The listing builds one solid part. Answer for the finished solid, in the listing's coordinates (mm). A direction names the side the tool comes from. Round coordinates to 2 decimals unless told otherwise and drop trailing zeros. Order: outer loops, then holes, each group sorted by start corner. A loop starts at its lowest first (then second) coordinate and runs counter-clockwise, first axis right, second up. Notation, with made-up numbers: (-39.5, 25.25) - (-27.5, 25.25) arc R15 ccw to (-27.5, 51.25) - close; hole circle Ø10 at (-4, 86). An arc over 180 degrees is marked (long way). Write item = value, one per line.
from build123d import *

# Parameters (mm, degrees)
BOSS_EXTRUDE1_DEPTH = 11
SKETCH2_R           = 35
CUT_EXTRUDE1_DEPTH  = 20
SKETCH3_R           = 14
BOSS_EXTRUDE2_DEPTH = 5
SKETCH4_R           = 10
CUT_EXTRUDE2_DEPTH  = 55
FILLET1_R           = 4
CHAMFER1_SIZE       = 2
SKETCH5_R           = 4
CUT_EXTRUDE3_DEPTH  = 10
SKETCH6_R           = 4
CUT_EXTRUDE4_DEPTH  = 31
SKETCH7_R           = 3
CUT_EXTRUDE5_DEPTH  = 6


with BuildPart() as part:
    # Sketch1 → Boss-Extrude1 (new body, symmetric)
    with BuildSketch(Plane.XY):
        with BuildLine():
            Line((-51.041834152, 0), (51.041834152, 0))
            Line((51.041834152, 0), (51.041834152, 10))
            Line((51.041834152, 10), (37, 10))
            ThreePointArc((37, 10), (34.171572875, 11.171572875), (33, 14))
            Line((33, 14), (33, 21.326056007))
            ThreePointArc((33, 21.326056007), (33.651668366, 24.876928527), (35.52173913, 27.965002788))
            ThreePointArc((35.52173913, 27.965002788), (47.48845464, 58.45277704), (36.877361169, 89.438440728))
            ThreePointArc((36.877361169, 89.438440728), (35.216671351, 92.397361701), (34.641016151, 95.741270355))
            Line((34.641016151, 95.741270355), (34.641016151, 107))
            Line((34.641016151, 107), (0, 107))
            ThreePointArc((0, 107), (-43.325294965, 78.972257605), (-35.52173913, 27.965002788))
            ThreePointArc((-35.52173913, 27.965002788), (-33.651668366, 24.876928527), (-33, 21.326056007))
            Line((-33, 21.326056007), (-33, 14))
            ThreePointArc((-33, 14), (-34.171572875, 11.171572875), (-37, 10))
            Line((-37, 10), (-51.041834152, 10))
            Line((-51.041834152, 10), (-51.041834152, 0))
        make_face()
    extrude(amount=BOSS_EXTRUDE1_DEPTH, both=True)

    # Sketch2 → Cut-Extrude1 (cut)
    with BuildSketch(Plane.XY.offset(11)):
        with Locations((0, 59.5)):
            Circle(SKETCH2_R)
    extrude(amount=-CUT_EXTRUDE1_DEPTH, mode=Mode.SUBTRACT)

    # Sketch3 → Boss-Extrude2 (add)
    with BuildSketch(Plane(origin=(0, 0, -11), x_dir=(-1, 0, 0), z_dir=(0, 0, -1))):
        with Locations((0, 59.5)):
            Circle(SKETCH3_R)
    extrude(amount=BOSS_EXTRUDE2_DEPTH)

    # Sketch4 → Cut-Extrude2 (cut)
    with BuildSketch(Plane(origin=(0, 0, -16), x_dir=(-1, 0, 0), z_dir=(0, 0, -1))):
        with Locations((0, 59.5)):
            Circle(SKETCH4_R)
    extrude(amount=-CUT_EXTRUDE2_DEPTH, mode=Mode.SUBTRACT)

    # Fillet1
    fillet1_edges = [part.edges().sort_by_distance(p)[0] for p in [
        (14, 59.5, -11),
    ]]
    fillet(fillet1_edges, radius=FILLET1_R)

    # Chamfer1
    chamfer1_edges = [part.edges().sort_by_distance(p)[0] for p in [
        (-51.041834152, 5, -11),
        (51.041834152, 5, -11),
        (51.041834152, 5, 11),
        (-51.041834152, 5, 11),
    ]]
    chamfer(chamfer1_edges, length=CHAMFER1_SIZE)

    # Sketch5 → Cut-Extrude3 (cut)
    with BuildSketch(Plane(origin=(0, 10, 0), x_dir=(1, 0, 0), z_dir=(0, 1, 0))):
        with Locations((-42, 0)):
            Circle(SKETCH5_R)
        with Locations((42, 0)):
            Circle(SKETCH5_R)
    extrude(amount=-CUT_EXTRUDE3_DEPTH, mode=Mode.SUBTRACT)

    # Sketch6 → Cut-Extrude4 (cut)
    with BuildSketch(Plane(origin=(0, 107, 0), x_dir=(1, 0, 0), z_dir=(0, 1, 0))):
        with Locations((26.861016151, 0)):
            Circle(SKETCH6_R)
    extrude(amount=-CUT_EXTRUDE4_DEPTH, mode=Mode.SUBTRACT)

    # Sketch7 → Cut-Extrude5 (cut)
    with BuildSketch(Plane.XY.offset(11)):
        with Locations((0, 99.5)):
            Circle(SKETCH7_R)
        with Locations((34.641016151, 79.5)):
            Circle(SKETCH7_R)
        with Locations((34.641016151, 39.5)):
            Circle(SKETCH7_R)
        with Locations((0, 19.5)):
            Circle(SKETCH7_R)
        with Locations((-34.641016151, 39.5)):
            Circle(SKETCH7_R)
        with Locations((-34.641016151, 79.5)):
            Circle(SKETCH7_R)
    extrude(amount=-CUT_EXTRUDE5_DEPTH, mode=Mode.SUBTRACT)


solid = part.part
Q1. Section B-B on z = 0 is taken. Determine the outline of the cut face in (x, y) (3 decimals), then the cut area to 3 significant figures.
Model answer:
outline = (-51.042, 0) - (-46, 0) - (-46, 10) - (-51.042, 10) - close; (-38, 0) - (38, 0) - (38, 10) - (37, 10) arc R4 cw to (33, 14) - (33, 21.326) arc R10 cw to (35.522, 27.965) arc R47.5 ccw to (36.877, 89.438) arc R10 cw to (34.641, 95.741) - (34.641, 107) - (30.861, 107) - (30.861, 76.011) arc R35 cw (long way) to (22.861, 86.002) - (22.861, 107) - (0, 107) arc R47.5 ccw to (-35.522, 27.965) arc R10 cw to (-33, 21.326) - (-33, 14) arc R4 cw to (-37, 10) - (-38, 10) - close; (46, 0) - (51.042, 0) - (51.042, 10) - (46, 10) - close
area = 4,480 mm^2
Q2. For faces 1 (the face through (10, 42, -11)), 2 (the face through (-33, 18, 0)), 3 (the face through (-35, 80, 5)), determine the directions among +Z, -Z, +X, -X, +Y, -Y from which every point of the face is accessible in a straight line to the end or side of a thin tool.
Model answer:
face_1 = -Z
face_2 = +Z, -Z, -X
face_3 = +Z
Q3. Section C-C on x = -42 is taken. Determine the outline of the cut face in (y, z).
Model answer:
outline = (0, -11) - (10, -11) - (10, -4) - (0, -4) - close; (0, 4) - (10, 4) - (10, 11) - (0, 11) - close; (37.31, -11) - (81.69, -11) - (81.69, 11) - (37.31, 11) - close
Q4. Flat-ended cylindrical pins translate along their axes: P1, Ø1.8, axis at x = 1, y = 100, coming from the +Z side; P2, Ø5.5, axis at x = 34.64, y = 39.5, coming from the -Z side; P3, Ø6, axis at x = -30, z = -3.5, coming from the +Y side; P4, Ø5, axis at x = 34, y = 38.5, coming from the +Z side. Find the tip coordinate at first contact, or state that the pin passes through.
Model answer:
P1 = 5
P2 = -11
P3 = 98.58
P4 = 11
Q5. Determine the mould class of faces 4 (the face through (-45.2, 5.1, 2.4)), 5 (the face through (34.203, 11.141, 0.154)), 6 (the face through (-35, 40, 5)) for opening direction Z: released by +Z, released by -Z, zero draft, split by the parting line, or undercut.
Model answer:
face_4 = undercut
face_5 = zero draft
face_6 = released by +Z
Q6. Find the intervals of material crossed by line 1 (X direction, y = 4, z = 0); line 2 (Y direction, x = 0, z = 8.2); line 3 (Z direction, x = 42, y = 7.5), in increasing order. Write a range as from..to.
Model answer:
line_1 = -51.04..-46, -38..38, 46..51.04
line_2 = 0..16.5, 22.5..24.5, 94.5..96.5, 102.5..107
line_3 = -11..-4, 4..11
Q7. Section D-D on y = 99.5 is taken. Determine the outline of the cut face in (x, z), then the cut area to 3 significant figures.
Model answer:
outline = (-25.62, -11) - (34.64, -11) - (34.64, 11) - (3, 11) - (3, 5) - (-3, 5) - (-3, 11) - (-25.62, 11) - close; hole circle Ø8 at (26.86, 0)
area = 1,240 mm^2
Q8. Section A-A on y = 59.5 is taken. Determine the outline of the cut face in (x, z), then the cut area to 3 significant figures.
Model answer:
outline = (-47.5, -11) - (-18, -11) arc R4 cw to (-14, -15) - (-14, -16) - (-10, -16) - (-10, -9) - (-35, -9) - (-35, 11) - (-47.5, 11) - close; (10, -16) - (14, -16) - (14, -15) arc R4 cw to (18, -11) - (47.5, -11) - (47.5, 11) - (35, 11) - (35, -9) - (10, -9) - close
area = 697 mm^2
